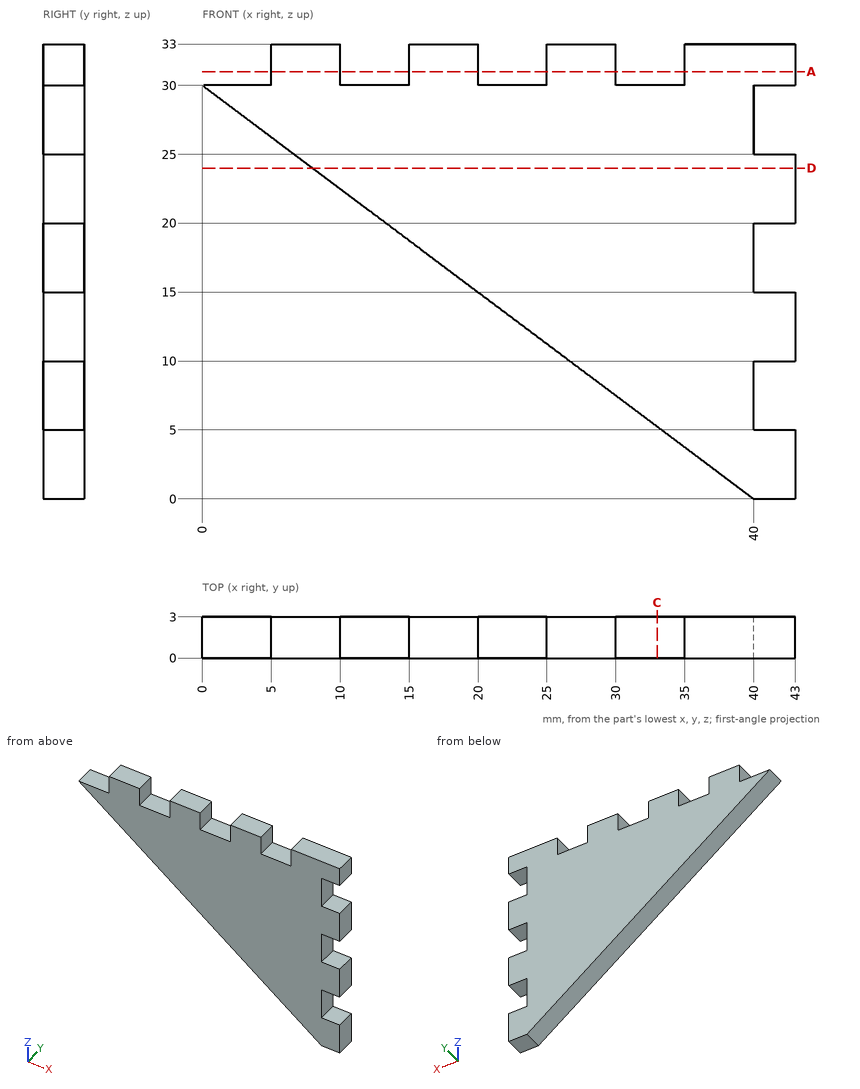
Geometry: see drawing. Coordinates: mm, zero at the bounding-box minimum. Give positions to 0.01 mm unless a question says otherwise; leave off trailing zeros. Loops run counter-clockwise (first coordinate to the right, second up) from the corner with the lowest first, then second, coordinate; pieces in that order, holes last. Notation, with made-up numbers: (85, -23.5) - (124, -23.5) arc R15 ccw to (124, -3.5) - close; hole circle Ø1 at (-0.5, 0.5). An arc over 180 degrees is marked (long way). Answer as CSV lines item,"result". Start each with the question number.
1. Ray query, L1, parallel to X at y = 0.4, z = 31.5; L2, parallel to Z at x = 40.5, y = 2.6; L3, parallel to Z at x = 29.5, y = 1.8 (3 decimals). Return the intervals inside material, ascending.
2. Section A-A, the plane z = 31. Return loops of the section in (x, y), plus the area to 3 significant figures.
3. Section C-C, the plane x = 33. Return loops of the section in (y, z), plus the area to 4 significant figures.
4. Pin query (flat end, axial travel): P1, Ø12, axis at x = 5.5, z = 14.5, coming from the +Y side; P2, Ø1, axis at y = 2, z = 11, coming from the -X side; P3, Ø1.5, axis at x = 2, y = 2, coming from the +Z side. Return the tip coordinate at first contact, or that it passes through.
5. Section D-D, the plane z = 24. Return loops of the section in (x, y), plus the area to 3 significant figures.
Answers:
1,L1,"x = 5 to 10, 15 to 20, 25 to 30, 35 to 43"
1,L2,"z = 0 to 5, 10 to 15, 20 to 25, 30 to 33"
1,L3,"z = 7.875 to 33"
2,outline,"(5, 0) - (10, 0) - (10, 3) - (5, 3) - close; (15, 0) - (20, 0) - (20, 3) - (15, 3) - close; (25, 0) - (30, 0) - (30, 3) - (25, 3) - close; (35, 0) - (43, 0) - (43, 3) - (35, 3) - close"
2,area,"69.0 mm2"
3,outline,"(0, 5.25) - (3, 5.25) - (3, 30) - (0, 30) - close"
3,area,"74.25 mm2"
4,P1,"passes through"
4,P2,"stops at x = 24.67"
4,P3,"stops at z = 30"
5,outline,"(8, 0) - (43, 0) - (43, 3) - (8, 3) - close"
5,area,"105 mm2"
